from build123d import *

# Parameters (mm, degrees)
SKETCH_1_R               = 54.5
EXTRUDE_1_DEPTH          = 4
SKETCH_2_W               = 100
SKETCH_2_H               = 35
CUT_EXTRUDE_1_DEPTH      = 4
FILLET_1_R               = 5
SKETCH_3_R               = 2.6
CUT_EXTRUDE_2_DEPTH      = 10
PATTERN_CIRCULAR_1_COUNT = 2
SKETCH_4_R               = 2.6
CUT_EXTRUDE_3_DEPTH      = 10
SKETCH_5_R               = 2.6
CUT_EXTRUDE_4_DEPTH      = 100
SKETCH_6_W               = 35.3
SKETCH_6_H               = 19.5
SKETCH_6_R               = 2.6
SKETCH_6_H_2             = 1.5
CUT_EXTRUDE_5_DEPTH      = 10
CUT_EXTRUDE_6_DEPTH      = 10
FILLET_2_R               = 1
SKETCH_8_W               = 35.3
SKETCH_8_H               = 3.1
CUT_EXTRUDE_7_DEPTH      = 10
SKETCH_10_W              = 35.3
SKETCH_10_H              = 4
CUT_EXTRUDE_8_DEPTH      = 54.5
SKETCH_11_R              = 56.5
SKETCH_11_R_2            = 54.5
EXTRUDE_2_DEPTH          = 4
SKETCH_12_W              = 3.5
SKETCH_12_H              = 5
CUT_EXTRUDE_9_DEPTH      = 6
PATTERN_CIRCULAR_2_COUNT = 2
SKETCH_14_W              = 102.88
SKETCH_14_H              = 30
CUT_EXTRUDE_10_DEPTH     = 30
FILLET_3_R               = 1
SKETCH_15_R              = 60
SKETCH_15_R_2            = 56.5
EXTRUDE_3_DEPTH          = 4


with BuildPart() as part:
    # 草图1 → 凸台-拉伸1 (new body)
    with BuildSketch(Plane(origin=(0, 0, 0), x_dir=(1, 0, 0), z_dir=(0, 1, 0))):
        with Locations(Location((0, 0, 0), (0, 0, 270))):
            Circle(SKETCH_1_R)
    extrude(amount=EXTRUDE_1_DEPTH)

    # 草图2 → 切除-拉伸1 (cut)
    with BuildSketch(Plane(origin=(0, 4, 0), x_dir=(1, 0, 0), z_dir=(0, 1, 0))):
        Rectangle(SKETCH_2_W, SKETCH_2_H)
    extrude(amount=-CUT_EXTRUDE_1_DEPTH, mode=Mode.SUBTRACT)

    # 圆角1
    fillet_1_edges = [part.edges().sort_by_distance(p)[0] for p in [
        (50, 2, -17.5),
        (50, 2, 17.5),
        (-50, 2, 17.5),
        (-50, 2, -17.5),
    ]]
    fillet(fillet_1_edges, radius=FILLET_1_R)

    # 草图3 → 切除-拉伸2 (cut)
    with BuildSketch(Plane.XZ):
        with Locations(Location((-23.75, 41.13620668, 0), (0, 0, 270))):
            Circle(SKETCH_3_R)
        with Locations(Location((23.75, 41.13620668, 0), (0, 0, 270))):
            Circle(SKETCH_3_R)
        with Locations(Location((0, 47.5, 0), (0, 0, 270))):
            Circle(SKETCH_3_R)
    cut_extrude_2 = extrude(amount=-CUT_EXTRUDE_2_DEPTH, mode=Mode.SUBTRACT)

    # 阵列(圆周)1: 切除-拉伸2 ×2 about axis
    pattern_circular_1_axis = Axis((0, 0, 0), (0, 1, 0))
    for i in range(1, PATTERN_CIRCULAR_1_COUNT):
        add(cut_extrude_2.rotate(pattern_circular_1_axis, i * 360 / PATTERN_CIRCULAR_1_COUNT), mode=Mode.SUBTRACT)

    # 草图4 → 切除-拉伸3 (cut)
    with BuildSketch(Plane.XZ):
        with Locations(Location((-15, 29.5, 0), (0, 0, 270))):
            Circle(SKETCH_4_R)
        with Locations(Location((15, 29.5, 0), (0, 0, 270))):
            Circle(SKETCH_4_R)
    extrude(amount=-CUT_EXTRUDE_3_DEPTH, mode=Mode.SUBTRACT)

    # 草图5 → 切除-拉伸4 (cut)
    with BuildSketch(Plane.XZ):
        with Locations(Location((-15, -33.5, 0), (0, 0, 270))):
            Circle(SKETCH_5_R)
        with Locations(Location((15, -33.5, 0), (0, 0, 270))):
            Circle(SKETCH_5_R)
    extrude(amount=-CUT_EXTRUDE_4_DEPTH, mode=Mode.SUBTRACT)

    # 草图6 → 切除-拉伸5 (cut)
    # profile 1 of 3: a face of its own
    with BuildSketch(Plane.XZ):
        with Locations((0, -27.25)):
            Rectangle(SKETCH_6_W, SKETCH_6_H)
        with Locations((-15, -33.5)):
            Circle(SKETCH_6_R, mode=Mode.SUBTRACT)
        with Locations((15, -33.5)):
            Circle(SKETCH_6_R, mode=Mode.SUBTRACT)
    # profile 2 of 3: a face of its own
    with BuildSketch(Plane.XZ):
        with Locations((0, -37.75)):
            Rectangle(SKETCH_6_W, SKETCH_6_H_2)
    # profile 3 of 3: a face of its own
    with BuildSketch(Plane.XZ):
        with Locations((0, 27.25)):
            Rectangle(SKETCH_6_W, SKETCH_6_H)
        with Locations((-15, 29.5)):
            Circle(SKETCH_6_R, mode=Mode.SUBTRACT)
        with Locations((15, 29.5)):
            Circle(SKETCH_6_R, mode=Mode.SUBTRACT)
    extrude(amount=-CUT_EXTRUDE_5_DEPTH, mode=Mode.SUBTRACT)

    # 草图7 → 切除-拉伸6 (cut)
    with BuildSketch(Plane.XZ):
        Polygon((-31, 22.5), (31, 22.5), (31, -22.5), (31, -29.4), (-31, -29.4), (-31, -22.5), align=None)
    extrude(amount=-CUT_EXTRUDE_6_DEPTH, mode=Mode.SUBTRACT)

    # 圆角2
    fillet_2_edges = [part.edges().sort_by_distance(p)[0] for p in [
        (31, 2, -17.5),
        (-31, 2, -17.5),
        (-31, 2, 17.5),
        (31, 2, 22.5),
        (31, 2, 17.5),
        (-31, 2, 22.5),
        (31, 2, -29.4),
        (-31, 2, -29.4),
    ]]
    fillet(fillet_2_edges, radius=FILLET_2_R)

    # 草图8 → 切除-拉伸7 (cut)
    with BuildSketch(Plane.XZ):
        with Locations((0, -40.05)):
            Rectangle(SKETCH_8_W, SKETCH_8_H)
    extrude(amount=-CUT_EXTRUDE_7_DEPTH, mode=Mode.SUBTRACT)

    # 草图10 → 切除-拉伸8 (cut)
    with BuildSketch(Plane.XZ):
        with Locations((0, 39)):
            Rectangle(SKETCH_10_W, SKETCH_10_H)
    extrude(amount=-CUT_EXTRUDE_8_DEPTH, mode=Mode.SUBTRACT)

    # 草图11 → 凸台-拉伸2 (add)
    with BuildSketch(Plane.XZ):
        with Locations(Location((0, 0, 0), (0, 0, 270))):
            Circle(SKETCH_11_R)
        Circle(SKETCH_11_R_2, mode=Mode.SUBTRACT)
    extrude(amount=-EXTRUDE_2_DEPTH)

    # 草图12 → 切除-拉伸9 (cut)
    with BuildSketch(Plane.XZ):
        with Locations((-8.25, 43.5)):
            Rectangle(SKETCH_12_W, SKETCH_12_H)
        with Locations((-11.75, 43.5)):
            Rectangle(SKETCH_12_W, SKETCH_12_H)
        with Locations((8.25, 43.5)):
            Rectangle(SKETCH_12_W, SKETCH_12_H)
        with Locations((11.75, 43.5)):
            Rectangle(SKETCH_12_W, SKETCH_12_H)
    cut_extrude_9 = extrude(amount=-CUT_EXTRUDE_9_DEPTH, mode=Mode.SUBTRACT)

    # 阵列(圆周)2: 切除-拉伸9 ×2 about axis
    pattern_circular_2_axis = Axis((0, 0, 0), (0, 1, 0))
    for i in range(1, PATTERN_CIRCULAR_2_COUNT):
        add(cut_extrude_9.rotate(pattern_circular_2_axis, i * 360 / PATTERN_CIRCULAR_2_COUNT), mode=Mode.SUBTRACT)

    # 草图14 → 切除-拉伸10 (cut)
    with BuildSketch(Plane(origin=(0, 0, 0), x_dir=(-1, 0, 0), z_dir=(0, -1, 0))):
        Rectangle(SKETCH_14_W, SKETCH_14_H)
    extrude(amount=-CUT_EXTRUDE_10_DEPTH, mode=Mode.SUBTRACT)

    # 圆角3
    fillet_3_edges = [part.edges().sort_by_distance(p)[0] for p in [
        (-49.330127019, 2, -15),
        (49.330127019, 2, 15),
        (-51.44, 2, 15),
        (-49.330127019, 2, 15),
        (51.44, 2, -15),
        (49.330127019, 2, -15),
        (-51.44, 2, -15),
        (51.44, 2, 15),
    ]]
    fillet(fillet_3_edges, radius=FILLET_3_R)

    # 草图15 → 凸台-拉伸3 (add)
    with BuildSketch(Plane.XZ):
        with Locations(Location((0, 0, 0), (0, 0, 270))):
            Circle(SKETCH_15_R)
        Circle(SKETCH_15_R_2, mode=Mode.SUBTRACT)
    extrude(amount=-EXTRUDE_3_DEPTH)


solid = part.part
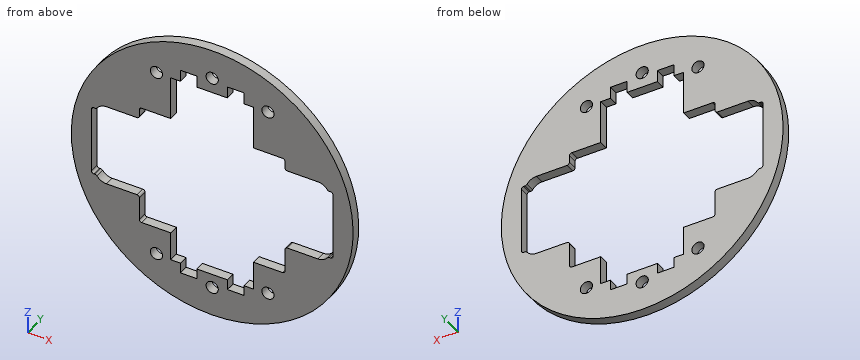
Geometry: final body of the model. Coordinates: model frame, mm. Coordinates: 2 decimals unless noted, no trailing zeros. Loops run counter-clockwise (first coordinate to the right, second up) from the corner with the lowest first, then second, coordinate; pieces in that order, holes last. Notation, with made-up numbers: (13, -38.5) - (72, -38.5) arc R16 cw to (72, -15.5) - close; hole circle Ø10 at (-11.75, -39.75). An arc over 180 degrees is marked (long way). Put each result on its own line as item: value. Start each with the question number.
Q1. Line query: line 1 (Z direction, x = -38.5, y = 2.2); line 2 (Z direction, x = -1, y = 1.55); line 3 (X direction, y = 2.6, z = -1.5). Output: solid intervals per line, ascending.
Q2. Cut plane C-C, the plane x = -15.5. Return loops of the section in (y, z).
Q3. Cut plane D-D, the plane y = 1.7. Give the number of separate pieces and of enclosed holes in the cut face, and give its area (3 significant figures).
Q4. Pin query (flat end, axial travel): pin 1 Ø1 at (x, y) = (-37, 3) entering from -Z; pin 2 Ø2 at (x, y) = (-23.5, 1) entering from -Z; pin 3 Ø2 at (y, z) = (1.5, 36) entering from -X; pin 4 Ø3 at (x, z) = (23.75, -41.14) entering from +Y. Return the tip coordinate at first contact, or that it passes through.
Q5. Cut plane B-B, the plane z = 0. Return loops of the section in (x, y).
Q6. Cut plane A-A, the plane x = 0. Return loops of the section in (y, z).
Filled sheet:
1. line 1: -46.02 to -17.5, 17.5 to 46.02
1. line 2: -59.99 to -49.9, -45.1 to -41.6, 41 to 45.1, 49.9 to 59.99
1. line 3: -59.98 to -51.44, 51.44 to 59.98
2. outline: (0, -57.96) - (4, -57.96) - (4, -41.6) - (0, -41.6) - close; (0, 41) - (4, 41) - (4, 57.96) - (0, 57.96) - close
3. separate pieces: 1
3. enclosed holes: 7
3. area: 5,350 mm²
4. pin 1: z = -47.62
4. pin 2: z = -55.62
4. pin 3: x = -48.73
4. pin 4: through
5. outline: (-60, 0) - (-51.44, 0) - (-51.44, 4) - (-60, 4) - close; (51.44, 0) - (60, 0) - (60, 4) - (51.44, 4) - close
6. outline: (0, -60) - (4, -60) - (4, -50.1) - (0, -50.1) - close; (0, -44.9) - (4, -44.9) - (4, -41.6) - (0, -41.6) - close; (0, 41) - (4, 41) - (4, 44.9) - (0, 44.9) - close; (0, 50.1) - (4, 50.1) - (4, 60) - (0, 60) - close
